from build123d import *

# Parameters (mm, degrees)
SKETCH1_W                = 650
SKETCH1_H                = 650
BOSS_EXTRUDE1_DEPTH      = 8
BOSS_EXTRUDE2_DEPTH      = 650
CUT_EXTRUDE2_DEPTH       = 921.277302922
CUT_EXTRUDE2_DEPTH_BACK  = 921.277302922
SKETCH4_R                = 11
CUT_EXTRUDE1_DEPTH       = 920.932062709
CUT_EXTRUDE1_DEPTH_BACK  = 920.932062709
SKETCH2_R                = 210
CUT_EXTRUDE3_DEPTH       = 921.277302998
CUT_EXTRUDE3_DEPTH_BACK  = 110
CUT_EXTRUDE4_DEPTH       = 110
CUT_EXTRUDE5_DEPTH       = 920.932062713
CUT_EXTRUDE5_DEPTH_BACK  = 920.932062713
SKETCH7_OUTSIDE_W        = 836.056
SKETCH7_OUTSIDE_H        = 836.056
BOSS_EXTRUDE3_DEPTH      = 160.08
BOSS_EXTRUDE4_DEPTH      = 160.08
SKETCH21_W               = 10
SKETCH21_H               = 4.3
CUT_EXTRUDE10_DEPTH      = 680.197320372
SKETCH22_W               = 10
SKETCH22_H               = 4.3
CUT_EXTRUDE11_DEPTH      = 278.189465889
BOSS_EXTRUDE5_DEPTH      = 60
CUT_EXTRUDE6_DEPTH       = 679.914574891
CUT_EXTRUDE6_DEPTH_BACK  = 679.914574891
SKETCH12_R               = 210
CUT_EXTRUDE14_DEPTH      = 11
SKETCH27_R               = 2.2
SKETCH27_R_2             = 2.75
CUT_EXTRUDE15_DEPTH      = 11
SKETCH28_R               = 2.75
CUT_EXTRUDE16_DEPTH      = 11
SKETCH29_W               = 20
SKETCH29_H               = 20
CUT_EXTRUDE17_DEPTH      = 10
CUT_EXTRUDE18_DEPTH      = 679.914574891
CUT_EXTRUDE18_DEPTH_BACK = 679.914574891
SKETCH30_W               = 195
SKETCH30_H               = 95
CUT_EXTRUDE19_DEPTH      = 589.600033979
CUT_EXTRUDE19_DEPTH_BACK = 589.600033979
SKETCH31_W               = 20.1
SKETCH31_H               = 20.1
SKETCH32_R               = 2.15
CUT_EXTRUDE20_DEPTH      = 10
CHAMFER1_SIZE            = 1


with BuildPart() as part:
    # Sketch1 → Boss-Extrude1 (new body)
    with BuildSketch(Plane(origin=(0, 0, 0), x_dir=(1, 0, 0), z_dir=(0, 1, 0))):
        with Locations((325, 325)):
            Rectangle(SKETCH1_W, SKETCH1_H)
    extrude(amount=BOSS_EXTRUDE1_DEPTH)

    # Sketch3 → Boss-Extrude2 (add)
    with BuildSketch(Plane.XY):
        Polygon((300, 43.707142143), (350, 43.707142143), (385, 8), (265, 8), align=None)
    extrude(amount=-BOSS_EXTRUDE2_DEPTH)

    # Sketch4 → Cut-Extrude2 (cut, two sides: drawn at the far end of the back side and taken through both)
    with BuildSketch(Plane.XY.offset(-CUT_EXTRUDE2_DEPTH_BACK)):
        with Locations((325, 22)):
            Circle(SKETCH4_R)
    extrude(amount=CUT_EXTRUDE2_DEPTH + CUT_EXTRUDE2_DEPTH_BACK, mode=Mode.SUBTRACT)

    # Sketch2 → Cut-Extrude1 (cut, two sides: drawn at the far end of the back side and taken through both)
    with BuildSketch(Plane(origin=(0, 8, 0), x_dir=(1, 0, 0), z_dir=(0, 1, 0)).offset(-CUT_EXTRUDE1_DEPTH_BACK)):
        with Locations(Location((325, 325, 0), (0, 0, 270))):
            Circle(SKETCH2_R)
    extrude(amount=CUT_EXTRUDE1_DEPTH + CUT_EXTRUDE1_DEPTH_BACK, mode=Mode.SUBTRACT)

    # Sketch5 → Cut-Extrude3 (cut, two sides: drawn at the far end of the back side and taken through both)
    with BuildSketch(Plane.XY.offset(-CUT_EXTRUDE3_DEPTH_BACK)):
        Polygon((300, 43.707142143), (350, 43.707142143), (365.396078824, 28), (350, 28), (350, 8), (300, 8), (300, 28), (284.603921176, 28), align=None)
    extrude(amount=CUT_EXTRUDE3_DEPTH + CUT_EXTRUDE3_DEPTH_BACK, mode=Mode.SUBTRACT)

    # Sketch6 → Cut-Extrude4 (cut)
    with BuildSketch(Plane(origin=(0, 0, -650), x_dir=(-1, 0, 0), z_dir=(0, 0, -1))):
        Polygon((-350, 43.707142143), (-300, 43.707142143), (-284.603921176, 28), (-300, 28), (-300, 8), (-350, 8), (-350, 28), (-365.396078824, 28), align=None)
    extrude(amount=-CUT_EXTRUDE4_DEPTH, mode=Mode.SUBTRACT)

    # Sketch7 outside → Cut-Extrude5 (cut, two sides: drawn at the far end of the back side and taken through both)
    with BuildSketch(Plane(origin=(0, 8, 0), x_dir=(1, 0, 0), z_dir=(0, 1, 0)).offset(-CUT_EXTRUDE5_DEPTH_BACK)):
        with Locations((325, 325)):
            Rectangle(SKETCH7_OUTSIDE_W, SKETCH7_OUTSIDE_H)
        Polygon((195, 455), (195, 489.924225025), (195, 650), (167.478198198, 686.544504505), (-70.838918919, 686.544504505), (-70.838918919, 472.462112512), (0, 455), (160.075774975, 455), align=None, mode=Mode.SUBTRACT)
    extrude(amount=CUT_EXTRUDE5_DEPTH + CUT_EXTRUDE5_DEPTH_BACK, mode=Mode.SUBTRACT)

    # Sketch8 → Boss-Extrude3 (add)
    with BuildSketch(Plane(origin=(0, 0, -650), x_dir=(-1, 0, 0), z_dir=(0, 0, -1))):
        Polygon((-195, 8), (-195, 28), (-185, 28), (-185, 17), (-175, 8), align=None)
    extrude(amount=-BOSS_EXTRUDE3_DEPTH)

    # Sketch10 → Boss-Extrude4 (add)
    with BuildSketch(Plane.ZY):
        Polygon((-455, 8), (-455, 28), (-465, 28), (-465, 17), (-475, 8), align=None)
    extrude(amount=-BOSS_EXTRUDE4_DEPTH)

    # Sketch21 → Cut-Extrude10 (cut, through all)
    with BuildSketch(Plane.ZY):
        with Locations((-460, 5)):
            Rectangle(SKETCH21_W, SKETCH21_H)
    extrude(amount=-CUT_EXTRUDE10_DEPTH, mode=Mode.SUBTRACT)

    # Sketch22 → Cut-Extrude11 (cut, through all)
    with BuildSketch(Plane(origin=(0, 0, -650), x_dir=(-1, 0, 0), z_dir=(0, 0, -1))):
        with Locations((-190, 5)):
            Rectangle(SKETCH22_W, SKETCH22_H)
    extrude(amount=-CUT_EXTRUDE11_DEPTH, mode=Mode.SUBTRACT)

    # Sketch23 → Boss-Extrude5 (add)
    with BuildSketch(Plane.XY.offset(-489.92)):
        Polygon((194.99464011, 8), (195, 28), (160.08, 28), (160.08, 8), align=None)
    extrude(amount=BOSS_EXTRUDE5_DEPTH)

    # Sketch12 → Cut-Extrude6 (cut, two sides: drawn at the far end of the back side and taken through both)
    with BuildSketch(Plane(origin=(0, 8, 0), x_dir=(1, 0, 0), z_dir=(0, 1, 0)).offset(-CUT_EXTRUDE6_DEPTH_BACK)):
        with Locations((325, 325)):
            Circle(SKETCH12_R)
    extrude(amount=CUT_EXTRUDE6_DEPTH + CUT_EXTRUDE6_DEPTH_BACK, mode=Mode.SUBTRACT)

    # Sketch26 → Cut-Extrude14 (cut)
    with BuildSketch(Plane(origin=(0, 28, 0), x_dir=(1, 0, 0), z_dir=(0, 1, 0))):
        Polygon((185, 489.92), (160.08, 489.92), (160.08, 465), align=None)
    extrude(amount=-CUT_EXTRUDE14_DEPTH, mode=Mode.SUBTRACT)

    # Sketch27 → Cut-Extrude15 (cut)
    with BuildSketch(Plane.ZY.offset(-185)):
        with Locations((-610, 23)):
            Circle(SKETCH27_R)
        with Locations((-570, 23)):
            Circle(SKETCH27_R)
        with Locations((-530, 23)):
            Circle(SKETCH27_R_2)
    extrude(amount=-CUT_EXTRUDE15_DEPTH, mode=Mode.SUBTRACT)

    # Sketch28 → Cut-Extrude16 (cut)
    with BuildSketch(Plane(origin=(0, 0, -465), x_dir=(-1, 0, 0), z_dir=(0, 0, -1))):
        with Locations((-120, 23)):
            Circle(SKETCH28_R)
        with Locations((-80, 23)):
            Circle(SKETCH28_R)
        with Locations((-40, 23)):
            Circle(SKETCH28_R)
    extrude(amount=-CUT_EXTRUDE16_DEPTH, mode=Mode.SUBTRACT)

    # Sketch29 → Cut-Extrude17 (cut)
    with BuildSketch(Plane(origin=(0, 8, 0), x_dir=(1, 0, 0), z_dir=(0, 1, 0))):
        with Locations((10, 640)):
            Rectangle(SKETCH29_W, SKETCH29_H)
    extrude(amount=-CUT_EXTRUDE17_DEPTH, mode=Mode.SUBTRACT)

    # Sketch30 → Cut-Extrude18 (cut, two sides: drawn at the far end of the back side and taken through both)
    with BuildSketch(Plane(origin=(0, 8, 0), x_dir=(1, 0, 0), z_dir=(0, 1, 0)).offset(-CUT_EXTRUDE18_DEPTH_BACK)):
        with Locations((97.5, 602.5)):
            Rectangle(SKETCH30_W, SKETCH30_H)
    extrude(amount=CUT_EXTRUDE18_DEPTH + CUT_EXTRUDE18_DEPTH_BACK, mode=Mode.SUBTRACT)

    # Sketch31 → Cut-Extrude19 (cut, two sides: drawn at the far end of the back side and taken through both)
    with BuildSketch(Plane(origin=(0, 8, 0), x_dir=(1, 0, 0), z_dir=(0, 1, 0)).offset(-CUT_EXTRUDE19_DEPTH_BACK)):
        with Locations((10.05, 544.95)):
            Rectangle(SKETCH31_W, SKETCH31_H)
    extrude(amount=CUT_EXTRUDE19_DEPTH + CUT_EXTRUDE19_DEPTH_BACK, mode=Mode.SUBTRACT)

    # Sketch32 → Cut-Extrude20 (cut)
    with BuildSketch(Plane(origin=(0, 8, 0), x_dir=(1, 0, 0), z_dir=(0, 1, 0))):
        with Locations(Location((50.1, 545, 0), (0, 0, 270))):
            Circle(SKETCH32_R)
        with Locations(Location((140.1, 545, 0), (0, 0, 270))):
            Circle(SKETCH32_R)
        with Locations(Location((10, 504.9, 0), (0, 0, 270))):
            Circle(SKETCH32_R)
    extrude(amount=-CUT_EXTRUDE20_DEPTH, mode=Mode.SUBTRACT)

    # Chamfer1
    chamfer1_edges = [part.edges().sort_by_distance(p)[0] for p in [
        (10, 8, -507.05),
        (140.1, 8, -547.15),
        (50.1, 8, -547.15),
    ]]
    chamfer(chamfer1_edges, length=CHAMFER1_SIZE)


solid = part.part
For this review, take the finished solid that the model builds, in its own axes (mm). A direction names the side the tool comes from. Round coordinates to 2 decimals unless told otherwise and drop trailing zeros. Loops run counter-clockwise (first coordinate to the right, second up) from the corner with the lowest first, then second, coordinate; pieces in that order, holes last. Notation, with made-up numbers: (-20, 1) - (-5, 1) arc R5 cw to (-5, 9) - close; hole circle Ø8 at (50, 37.5). An arc over 180 degrees is marked (long way). One line per item, written item: value. Start each with the question number.
Item 1: For L1, parallel to X at y = 5, z = -545; L2, parallel to Y at x = 120, z = -458; L3, parallel to Y at x = 70, z = -486, list the stretches that pass through material, from the lowest coordinate up.
Item 2: Take a section at B-B (z = -545). Give the boundary of the cut face in (x, y), plus the area to 3 significant figures.
Item 3: For faces 1 (the flat face through (83, 2.85, -460)), 2 (the flat face through (190, 7.15, -519)), 3 (the flat face through (10, 4, -534.9)), 4 (the flat face through (185, 23, -523)), 5 (the cylindrical face through (42.747, 23.121, -460.07)), list the 3-axis set-ups (+Z, -Z, +X, -X, +Y, -Y) from which the entire face can be reached by the end or side of a thin tool; tool diameter is ignored.
Item 4: The part is to be moulded in two halves that separate along Y. For faces 6 (the flat face through (170, 13, -489.92)), 7 (the flat face through (96, 0, -506)), 8 (the flat face through (83, 5, -465)), 9 (the cylindrical face through (120.358, 25.727, -460.07)), say which applies: +Y half, -Y half, draft (parallel to the pull), parting line (faces both ways), or undercut.
Item 5: Take a section at A-A (x = 140.1). Give the boundary of the cut face in (y, z).
Item 6: Take a section at D-D (y = 23). Give the boundary of the cut face in (x, z).
Item 7: Clearance check with flat-ended pins moving along their axes: pin 1 Ø2 at (y, z) = (5, -515.5) entering from +X; pin 2 Ø12 at (y, z) = (22, -503.5) entering from -X; pin 3 Ø3.5 at (x, y) = (40, 23) entering from +Z; pin 4 Ø5 at (x, y) = (139, 15) entering from -Z. State where each tip first meets the part, or that it passes through.
Item 8: Take a section at C-C (z = -530). Give the boundary of the cut face in (x, y).
Answer below:
1. L1: x = 20.1 to 47.95, 52.25 to 137.95, 142.25 to 185
1. L2: y = 0 to 2.85, 7.15 to 20.25, 25.75 to 28
1. L3: y = 0 to 8
2. outline: (20.1, 0) - (47.95, 0) - (47.95, 7) - (46.95, 8) - (20.1, 8) - close; (52.25, 0) - (137.95, 0) - (137.95, 7) - (136.95, 8) - (53.25, 8) - (52.25, 7) - close; (142.25, 0) - (195, 0) - (195, 2.85) - (185, 2.85) - (185, 7.15) - (195, 7.15) - (195, 28) - (185, 28) - (185, 17) - (175, 8) - (143.25, 8) - (142.25, 7) - close
2. area: 1,530 mm2
3. face 1: +Z, +X, -X
3. face 2: +Z, -Z, +X
3. face 3: -Z, -X, +Y, -Y
3. face 4: -Z, -X, +Y
3. face 5: +Z, -Z
4. face 6: draft
4. face 7: -Y half
4. face 8: undercut
4. face 9: undercut
5. outline: (0, -555) - (8, -555) - (8, -548.15) - (7, -547.15) - (0, -547.15) - close; (0, -542.85) - (7, -542.85) - (8, -541.85) - (8, -475) - (17, -465) - (28, -465) - (28, -455) - (7.15, -455) - (7.15, -465) - (2.85, -465) - (2.85, -455) - (0, -455) - close
6. outline: (0, -465) - (37.25, -465) - (37.25, -455) - (0, -455) - close; (42.75, -465) - (77.25, -465) - (77.25, -455) - (42.75, -455) - close; (82.75, -465) - (117.25, -465) - (117.25, -455) - (82.75, -455) - close; (122.75, -465) - (160.08, -465) - (185, -489.92) - (185, -527.25) - (195, -527.25) - (195, -489.92) arc R210 cw to (160.08, -455) - (122.75, -455) - close; (185, -555) - (195, -555) - (195, -532.75) - (185, -532.75) - close
7. pin 1: stops at x = 185
7. pin 2: stops at x = 183.89
7. pin 3: passes through
7. pin 4: stops at z = -470
8. outline: (0, 0) - (195, 0) - (195, 2.85) - (185, 2.85) - (185, 7.15) - (195, 7.15) - (195, 20.25) - (185, 20.25) - (185, 17) - (175, 8) - (0, 8) - close; (185, 25.75) - (195, 25.75) - (195, 28) - (185, 28) - close
